from build123d import *

# Parameters (mm, degrees)
F1_DEPTH = 10


with BuildPart() as f1:
    # F0 (on Front) → F1 (new body)
    with BuildSketch(Plane.XZ):
        with BuildLine():
            Line((-100, 0), (-20.000535, 0))
            ThreePointArc((-20.000535, 0), (-0.000535, 20), (-20.000535, 40))
            Line((-20.000535, 40), (-100, 40))
            Line((-100, 40), (-100, 0))
        make_face()
        with BuildLine():
            ThreePointArc((-70.246651, 17.5), (-89.995429, 19.404993), (-70.397874, 22.5))
            Line((-70.397874, 22.5), (-68.087297, 22.5))
            Line((-68.087297, 22.5), (-68.087297, 17.5))
            Line((-68.087297, 17.5), (-70.246651, 17.5))
        make_face(mode=Mode.SUBTRACT)
    extrude(amount=F1_DEPTH)


solid = f1.part
Verification items for the finished model (mm, model axes). A direction names the side the tool comes from. Give positions to 0.01 mm unless a question says otherwise; leave off trailing zeros. Write each loop counter-clockwise with the first axis right and the second up, starting at its lowest first coordinate (ties: lowest second). Pieces come first, ordered by that corner, then holes.
(1) Access from +Z, -Z, +X, -X, +Y, -Y to the whole of each face (thin tool, end or side, straight path). Record for faces 5 (the face through (0, -5, 20)), 6 (the face through (-69, -5, 17.5)).
(2) Cross-section at B-B (z = 16). Enter the section's corners in (x, y).
(3) Material ranges on line 1 (Z direction, x = -80, y = -4); line 2 (Z direction, x = -86, y = -2.5); line 3 (X direction, y = -4.75, z = 13.5), recorded low to high.
(4) Cross-section at A-A (y = -2.5). Enter the section's corners in (x, z).
(5) Cross-section at C-C (x = -80). Enter the section's corners in (y, z), plus the area to 3 significant figures.
(6) Cross-section at D-D (z = 33.5). Enter the section's corners in (x, y), plus the area to 3 significant figures.
(7) Mould release check, pull along Z, two halves, no side actions. Record for faces 1 (the face through (-69, -5, 22.5)), 2 (the face through (-59, -5, 40)), 3 (the face through (-68.087, -5, 20)), 4 (the face through (-51, 0, 20)): +Z half, -Z half, draft (parallel to the pull), parting line (faces both ways), or undercut.
Worked out:
1. face 5: +X, +Y, -Y
1. face 6: +Y, -Y
2. outline: (-100, -10) - (-89.29, -10) - (-89.29, 0) - (-100, 0) - close; (-70.71, -10) - (-0.4, -10) - (-0.4, 0) - (-70.71, 0) - close
3. line 1: z = 0 to 9.71, 29.71 to 40
3. line 2: z = 0 to 11.71, 27.71 to 40
3. line 3: x = -100 to -87.84, -72.16 to -1.09
4. outline: (-100, 0) - (-20, 0) arc R20 ccw to (-20, 40) - (-100, 40) - close; hole (-70.4, 22.5) arc R10 ccw (long way) to (-70.25, 17.5) - (-68.09, 17.5) - (-68.09, 22.5) - close
5. outline: (-10, 0) - (0, 0) - (0, 9.71) - (-10, 9.71) - close; (-10, 29.71) - (0, 29.71) - (0, 40) - (-10, 40) - close
5. area: 200 mm2
6. outline: (-100, -10) - (-5.24, -10) - (-5.24, 0) - (-100, 0) - close
6. area: 948 mm2
7. face 1: undercut
7. face 2: +Z half
7. face 3: undercut
7. face 4: draft
